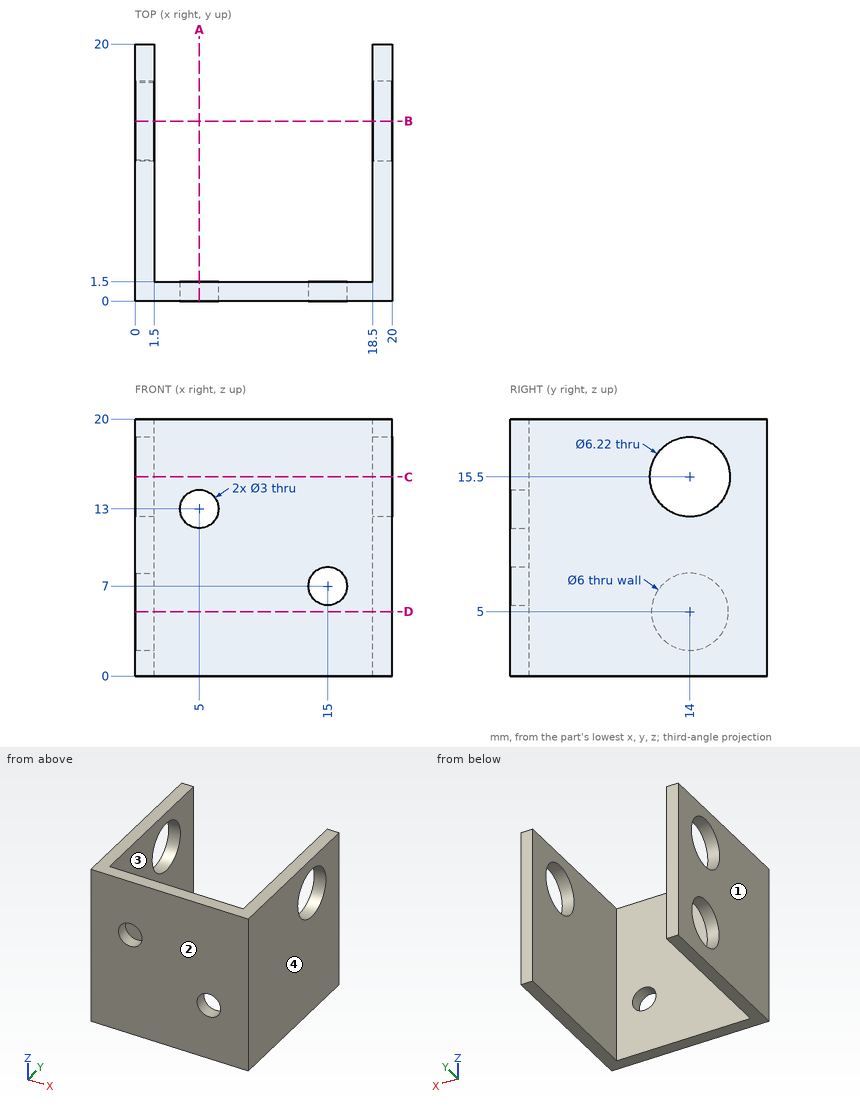
Print and shaded views of the part. All mm, measured from the part's lowest x, y and z. Round coordinates to 2 decimals unless told otherwise and drop trailing zeros. Write each loop counter-clockwise with the first axis right and the second up, starting at its lowest first coordinate (ties: lowest second). Pieces come first, ordered by that corner, then holes. Notation, with made-up numbers: (63, 77) -> (102, 77) arc R9 cw to (102, 85) -> close; hole circle Ø4 at (54, 20.25). An arc over 180 degrees is marked (long way). Answer in a Markdown table with one row per item. Add a question column.
Item 1: Saw through at C-C, the plane z = 15.5. Write the cut outline in (x, y), then the cut area to 3 significant figures.
Item 2: Mould opens along X. For the marked faces 1, 2, 3 and 4 say: pulls with the +X half, pulls with the -X half, needs draft (parallel to the pull), parting line crosses it, or undercut.
Item 3: Saw through at B-B, the plane y = 14. Write the cut outline in (x, z), then the cut area to 3 significant figures.
Item 4: Saw through at A-A, the plane x = 5. Write the cut outline in (y, z).
Item 5: Drill centre lines: line 1 (X direction, y = 3.75, z = 12); line 2 (Z direction, x = 5, y = 0.5); line 3 (Y direction, x = 19.55, z = 15.5). Where is each one in solid material? Low to high. Write a range as from..to.
Item 6: Drop flat-ended pins along their axis: pin 1 Ø5 at (x, z) = (8.5, 12) entering from +Y; pin 2 Ø5 at (y, z) = (14, 5) entering from -X. Give the stop position or say it passes through.
Item 7: Saw through at D-D, the plane z = 5. Write the cut outline in (x, y).
Findings below:
| question | item | result |
|---|---|---|
| 1 | outline | (0, 0) -> (20, 0) -> (20, 10.89) -> (18.5, 10.89) -> (18.5, 1.5) -> (1.5, 1.5) -> (1.5, 10.89) -> (0, 10.89) -> close; (0, 17.11) -> (1.5, 17.11) -> (1.5, 20) -> (0, 20) -> close; (18.5, 17.11) -> (20, 17.11) -> (20, 20) -> (18.5, 20) -> close |
| 1 | area | 66.8 mm^2 |
| 2 | face 1 | pulls with the -X half |
| 2 | face 2 | needs draft |
| 2 | face 3 | undercut |
| 2 | face 4 | pulls with the +X half |
| 3 | outline | (0, 0) -> (1.5, 0) -> (1.5, 2) -> (0, 2) -> close; (0, 8) -> (1.5, 8) -> (1.5, 12.39) -> (0, 12.39) -> close; (0, 18.61) -> (1.5, 18.61) -> (1.5, 20) -> (0, 20) -> close; (18.5, 0) -> (20, 0) -> (20, 12.39) -> (18.5, 12.39) -> close; (18.5, 18.61) -> (20, 18.61) -> (20, 20) -> (18.5, 20) -> close |
| 3 | area | 32.3 mm^2 |
| 4 | outline | (0, 0) -> (1.5, 0) -> (1.5, 11.5) -> (0, 11.5) -> close; (0, 14.5) -> (1.5, 14.5) -> (1.5, 20) -> (0, 20) -> close |
| 5 | line 1 | x = 0..1.5, 18.5..20 |
| 5 | line 2 | z = 0..11.5, 14.5..20 |
| 5 | line 3 | y = 0..10.89, 17.11..20 |
| 6 | pin 1 | stops at y = 1.5 |
| 6 | pin 2 | stops at x = 18.5 |
| 7 | outline | (0, 0) -> (20, 0) -> (20, 20) -> (18.5, 20) -> (18.5, 1.5) -> (1.5, 1.5) -> (1.5, 11) -> (0, 11) -> close; (0, 17) -> (1.5, 17) -> (1.5, 20) -> (0, 20) -> close |
